from build123d import *

# Parameters (mm, degrees)
F1_DEPTH  = 88.9
F0_W      = 110.728125
F0_H      = 41.671875
F2_DEPTH  = 3.175
F3_W      = 9.525
F3_H      = 3.175
F4_DEPTH  = 88.9
F5_W      = 9.525
F5_H      = 22.86
F6_DEPTH  = 3.175
F8_DEPTH  = 4.7625
F9_R      = 9.525
F10_W     = 49.53
F10_H     = 26.924
F10_R     = 1.778
F11_DEPTH = 4.7625
F12_DEPTH = 1.905
F14_DEPTH = 4.7625
F15_R     = 9.525
F16_DEPTH = 4.7625


with BuildPart() as f1:
    # F0 (on Top) → F1 (new body)
    with BuildSketch(Plane.XY):
        Polygon((0, 46.434375), (0, 0), (4.7625, 0), (4.7625, 41.671875), (115.490625, 41.671875), (115.490625, 0), (120.253125, 0), (120.253125, 46.434375), align=None)
    extrude(amount=F1_DEPTH)

    # F0 (on Top) → F2 (join)
    with BuildSketch(Plane.XY):
        Polygon((0, 46.434375), (0, 0), (4.7625, 0), (4.7625, 41.671875), (115.490625, 41.671875), (115.490625, 0), (120.253125, 0), (120.253125, 46.434375), align=None)
        with Locations((60.1265625, 20.8359375)):
            Rectangle(F0_W, F0_H)
    extrude(amount=-F2_DEPTH)

    # F3 (on face) → F4 (join, through all)
    with BuildSketch(Plane.XY):
        with Locations((110.728125, 8.73125)):
            Rectangle(F3_W, F3_H)
    extrude(amount=F4_DEPTH)

    # F5 (on face) → F6 (cut, through all)
    with BuildSketch(Plane.XZ.offset(-7.14375)):
        with Locations((110.728125, 77.4700000001)):
            Rectangle(F5_W, F5_H)
        with BuildLine():
            Line((112.315625, 58.4993750001), (112.315625, 61.6743750001))
            ThreePointArc((112.315625, 61.6743750001), (110.728125, 63.2618750001), (109.140625, 61.6743750001))
            Line((109.140625, 61.6743750001), (109.140625, 58.4993750001))
            ThreePointArc((109.140625, 58.4993750001), (110.728125, 56.9118750001), (112.315625, 58.4993750001))
        make_face()
    extrude(amount=-F6_DEPTH, mode=Mode.SUBTRACT)

    # F7 (on face) → F8 (cut, through all)
    with BuildSketch(Plane(origin=(0, 0, 0), x_dir=(0, -1, 0), z_dir=(-1, 0, 0))):
        with BuildLine():
            Line((-23.01875, 66.278125), (-23.01875, 78.978125))
            ThreePointArc((-23.01875, 78.978125), (-24.60625, 80.565625), (-26.19375, 78.978125))
            Line((-26.19375, 78.978125), (-26.19375, 66.278125))
            ThreePointArc((-26.19375, 66.278125), (-24.60625, 64.690625), (-23.01875, 66.278125))
        make_face()
    extrude(amount=-F8_DEPTH, mode=Mode.SUBTRACT)

    # F9
    f9_edges = [f1.edges().sort_by_distance(p)[0] for p in [
        (120.253125, 46.434375, 42.8625),
        (0, 46.434375, 42.8625),
    ]]
    fillet(f9_edges, radius=F9_R)

    # F10 (on face) → F11 (cut, through all)
    with BuildSketch(Plane(origin=(0, 46.434375, 0), x_dir=(-1, 0, 0), z_dir=(0, 1, 0))):
        with Locations((-62.6407308385, 25.0270083303)):
            Rectangle(F10_W, F10_H)
        with Locations((-64.0885308385, 45.1438083303)):
            Circle(F10_R)
        with Locations((-64.0885308385, 5.1642083303)):
            Circle(F10_R)
    extrude(amount=-F11_DEPTH, mode=Mode.SUBTRACT)

    # F10 (on face) → F12 (cut)
    with BuildSketch(Plane(origin=(0, 46.434375, 0), x_dir=(-1, 0, 0), z_dir=(0, 1, 0))):
        Polygon((-94.3145308385, 38.4890083303), (-94.3145308385, 11.5650083303), (-64.0885308385, 0.6430083303), (-34.6245308385, 11.5650083303), (-34.6245308385, 38.4890083303), (-64.0885308385, 49.6650083303), align=None)
        with Locations((-64.0885308385, 5.1642083303)):
            Circle(F10_R, mode=Mode.SUBTRACT)
        with Locations((-62.6407308385, 25.0270083303)):
            Rectangle(F10_W, F10_H, mode=Mode.SUBTRACT)
        with Locations((-64.0885308385, 45.1438083303)):
            Circle(F10_R, mode=Mode.SUBTRACT)
    extrude(amount=-F12_DEPTH, mode=Mode.SUBTRACT)

    # F13 (on face) → F14 (cut, through all)
    with BuildSketch(Plane.XZ.offset(-41.671875)):
        with BuildLine():
            Line((113.903125, 58.4993750001), (113.903125, 61.6743750001))
            ThreePointArc((113.903125, 61.6743750001), (110.728125, 64.8493750001), (107.553125, 61.6743750001))
            Line((107.553125, 61.6743750001), (107.553125, 58.4993750001))
            ThreePointArc((107.553125, 58.4993750001), (110.728125, 55.3243750001), (113.903125, 58.4993750001))
        make_face()
    extrude(amount=-F14_DEPTH, mode=Mode.SUBTRACT)

    # F15 (on face) → F16 (cut, through all)
    with BuildSketch(Plane.YZ.offset(120.253125)):
        with Locations((24.6292781085, 16.2439811975)):
            Circle(F15_R)
    extrude(amount=-F16_DEPTH, mode=Mode.SUBTRACT)


solid = f1.part
The model under review builds one solid part; all positions refer to its coordinate system, in mm. A direction names the side the tool comes from. Round coordinates to 2 decimals unless told otherwise and drop trailing zeros. Write each loop counter-clockwise with the first axis right and the second up, starting at its lowest first coordinate (ties: lowest second). Pieces come first, ordered by that corner, then holes. Notation, with made-up numbers: M 24,11.25 L 37,11.25 A23 ccw 37,28.25 Z; hole C -23.75,22 d4. An arc over 180 degrees is marked long. Answer as CSV lines item,"result". Start each with the question number.
Q1. The part is to be moulded in two halves that separate along X. For faces 4 (the face through (87.406, 43, 25)), 5 (the face through (0, 19, 44)), 6 (the face through (49.56, 45.5, 6.03)), 7 (the face through (2, 26.194, 73)), say which applies: +X half, -X half, draft (parallel to the pull), parting line (faces both ways), or undercut.
Q2. Clearance check with flat-ended pins moving along their axes: P1, Ø0.6, axis at y = 45.5, z = 27, coming from the -X side; P2, Ø6, axis at x = 66.5, z = 35, coming from the +Y side; P3, Ø2.5, axis at y = 43, z = 59.5, coming from the +X side; P4, Ø3, axis at y = 41, z = 69.5, coming from the +X side. State where each tip first meets the part, or that it passes through.
Q3. Consider section B-B, the plane y = 24.5. Give the boundary of the cut face in (x, z) (1 decimal).
Q4. Wall thickness on line 1 along Y through (x, z) = (107.5, 63); line 2 along X through (y, z) = (2, 42); line 3 along X through (y, z) = (37.5, 64): over which ranges is each line inside the solid? List them lowest first.
Q5. Consider section C-C, the plane x = 57. Give the boundary of the cut face in (y, z) (3 decimals), then the cut area to 3 significant figures.
Q6. Consider section D-D, the plane y = 13.5. Give the boundary of the cut face in (x, z) (1 decimal), then the cut area to 3 significant figures.
Q7. Tool access review of faces 1 (the face through (112.316, 9, 60)), 2 (the face through (49.15, 45.5, 44)), 3 (the face through (117.905, 15.113, 16.663)): name each direction out of +Z, -Z, +X, -X, +Y, -Y from which nothing blocks a thin tool from reaching the whole face with its end or side.
Result set:
1,face 4,"undercut"
1,face 5,"-X half"
1,face 6,"undercut"
1,face 7,"draft"
2,P1,"stops at x = 4.84"
2,P2,"passes through"
2,P3,"stops at x = 118.93"
2,P4,"stops at x = 119.89"
3,outline,"M 0,-3.2 L 120.3,-3.2 L 120.3,6.7 L 115.5,6.7 L 115.5,0 L 4.8,0 L 4.8,64.7 L 0,64.7 Z; M 0,80.6 L 4.8,80.6 L 4.8,88.9 L 0,88.9 Z; M 115.5,25.8 L 120.3,25.8 L 120.3,88.9 L 115.5,88.9 Z"
4,line 1,"y = 7.14 to 10.32, 41.67 to 46.43"
4,line 2,"x = 0 to 4.76, 115.49 to 120.25"
4,line 3,"x = 0.02 to 4.76, 115.49 to 120.23"
5,outline,"M 0,-3.175 L 46.434,-3.175 L 46.434,3.271 L 44.529,3.271 L 44.529,11.565 L 41.672,11.565 L 41.672,0 L 0,0 Z; M 41.672,38.489 L 44.529,38.489 L 44.529,46.976 L 46.434,46.976 L 46.434,88.9 L 41.672,88.9 Z"
5,area,"411 mm²"
6,outline,"M 0,-3.2 L 120.3,-3.2 L 120.3,88.9 L 115.5,88.9 L 115.5,0 L 4.8,0 L 4.8,88.9 L 0,88.9 Z"
6,area,"1,230 mm²"
7,face 1,"+Y, -Y"
7,face 2,"+Y"
7,face 3,"+X"
